Input: part model. Units: mm. Frame: model coordinates. Round coordinates to 2 decimals unless told otherwise and drop trailing zeros. Loops run counter-clockwise (first coordinate to the right, second up) from the corner with the lowest first, then second, coordinate; pieces in that order, holes last. Notation, with made-up numbers: (72, 9.5) -> (102, 9.5) arc R30 cw to (102, 46.5) -> close; hole circle Ø5 at (11.5, 36). An arc over 180 degrees is marked (long way). One line per question, with ' | ' between items. Start each with the question number.
Q1. Material intervals for L1, parallel to Y at x = 0, z = 3.45; L2, parallel to X at y = 1.5, z = 3.9; L3, parallel to Y at x = -1.25, z = 4, sorted ascending.
Q2. Cut plane D-D on y = 9. Return loops of the section in (x, z), and give its area (3 significant figures).
Q3. Mould query, pull axis X, two halves, no side actions, for faces 1 (the face through (-11.248, 0.099, 2.465)), 2 (the face through (3, -3, 5)), 3 (the face through (11.923, 3.755, 2.465)). Classes: pulls with the +X half, pulls with the -X half, needs draft (parallel to the pull), parting line crosses it, or undercut.
Q4. Cut plane B-B on x = 9.25. Return loops of the section in (y, z).
Q5. Cut plane C-C on z = 2.7. Return loops of the section in (x, y).
Q6. Contact query for flat-ended pins moving along their axis: P1, Ø5, axis at x = 0, y = 9, coming from the +Z side; P2, Ø2, axis at x = -2, z = 4, coming from the +Y side; P3, Ø4, axis at x = 0, y = -9, coming from the -Z side. Output: stop coordinate, or through.
Q7. Cut plane A-A on y = 0. Return loops of the section in (x, z).
from build123d import *

# Parameters (mm, degrees)
F0_R     = 12.5
F0_R_2   = 3
F1_DEPTH = 5
F2_R     = 2.25
F3_DEPTH = 10
F4_R     = 2.25
F5_DEPTH = 10


with BuildPart() as f1:
    # F0 (on Top) → F1 (new body)
    with BuildSketch(Plane.XY):
        Circle(F0_R)
        Circle(F0_R_2, mode=Mode.SUBTRACT)
    extrude(amount=F1_DEPTH)

    # F2 (on Top) → F3 (cut)
    with BuildSketch(Plane.XY):
        with Locations((0, 9)):
            Circle(F2_R)
        with Locations((0, -9)):
            Circle(F2_R)
    extrude(amount=F3_DEPTH, mode=Mode.SUBTRACT)

    # F4 (on Top) → F5 (cut)
    with BuildSketch(Plane.XY):
        with Locations((-9, 0)):
            Circle(F4_R)
        with Locations((9, 0)):
            Circle(F4_R)
    extrude(amount=F5_DEPTH, mode=Mode.SUBTRACT)


solid = f1.part
Results:
1) L1: -12.5 to -11.25, -6.75 to -3, 3 to 6.75, 11.25 to 12.5 | L2: -12.41 to -10.68, -7.32 to -2.6, 2.6 to 7.32, 10.68 to 12.41 | L3: -12.44 to -10.87, -7.13 to -2.73, 2.73 to 7.13, 10.87 to 12.44
2) outline: (-8.67, 0) -> (-2.25, 0) -> (-2.25, 5) -> (-8.67, 5) -> close; (2.25, 0) -> (8.67, 0) -> (8.67, 5) -> (2.25, 5) -> close | area: 64.2 mm^2
3) face 1: undercut | face 2: needs draft | face 3: parting line crosses it
4) outline: (-8.41, 0) -> (-2.24, 0) -> (-2.24, 5) -> (-8.41, 5) -> close; (2.24, 0) -> (8.41, 0) -> (8.41, 5) -> (2.24, 5) -> close
5) outline: circle Ø25 at (0, 0); hole circle Ø4.5 at (-9, 0); hole circle Ø6 at (0, 0); hole circle Ø4.5 at (0, -9); hole circle Ø4.5 at (0, 9); hole circle Ø4.5 at (9, 0)
6) P1: z = 5 | P2: y = 12.46 | P3: through
7) outline: (-12.5, 0) -> (-11.25, 0) -> (-11.25, 5) -> (-12.5, 5) -> close; (-6.75, 0) -> (-3, 0) -> (-3, 5) -> (-6.75, 5) -> close; (3, 0) -> (6.75, 0) -> (6.75, 5) -> (3, 5) -> close; (11.25, 0) -> (12.5, 0) -> (12.5, 5) -> (11.25, 5) -> close
